Design review of the part built by this model. Coordinates are the model's own, in mm. A direction names the side the tool comes from. Give positions to 0.01 mm unless a question says otherwise; leave off trailing zeros. Order: outer loops, then holes, each group sorted by start corner. A loop starts at its lowest first (then second) coordinate and runs counter-clockwise, first axis right, second up. Notation, with made-up numbers: M 89.25,-26 L 99.25,-26 A14 ccw 99.25,0 Z; hole C 86.25,-30 d6. An arc over 180 degrees is marked long. Answer as a JSON object with one key per item and string values.
from build123d import *

# Parameters (mm, degrees)
SKETCH1_W            = 1094.236516538
SKETCH1_H            = 400
BOSS_EXTRUDE1_DEPTH  = 18
CAVITY1_START        = -15
CAVITY1_OUTLINE_W    = 18
CAVITY1_OUTLINE_H    = 18
CAVITY1_DEPTH        = 30
CAVITY1_START_2      = 813.236516538
CAVITY1_2_OUTLINE_W  = 18
CAVITY1_2_OUTLINE_H  = 18
CAVITY1_2_DEPTH      = 30
CAVITY1_START_3      = 389.118258269
CAVITY1_3_OUTLINE_W  = 18
CAVITY1_3_OUTLINE_H  = 18
CAVITY1_3_DEPTH      = 50
CAVITY1_START_4      = -35
CAVITY1_4_OUTLINE_W  = 18
CAVITY1_4_OUTLINE_H  = 18
CAVITY1_4_DEPTH      = 20
CAVITY1_START_5      = 15
CAVITY1_5_OUTLINE_W  = 18
CAVITY1_5_OUTLINE_H  = 18
CAVITY1_5_DEPTH      = 20
CAVITY1_START_6      = 793.236516538
CAVITY1_6_OUTLINE_W  = 18
CAVITY1_6_OUTLINE_H  = 18
CAVITY1_6_DEPTH      = 20
CAVITY1_START_7      = 843.236516538
CAVITY1_7_OUTLINE_W  = 18
CAVITY1_7_OUTLINE_H  = 18
CAVITY1_7_DEPTH      = 20
SKETCH2_W            = 18
SKETCH2_H            = 50
CUT_EXTRUDE1_DEPTH   = 987.255362837
SKETCH3_W            = 798.236516538
SKETCH3_H            = 209.4
CUT_EXTRUDE2_DEPTH   = 18
SKETCH4_W            = 734.236516538
SKETCH4_H            = 110.6
CUT_EXTRUDE3_DEPTH   = 20
M3_CLEARANCE_HOLE1_D = 3.4
SKETCH7_R            = 3
CUT_EXTRUDE4_DEPTH   = 30


# Read off the part's stored shape, not the designer's step: Cavity1
with BuildPart() as part:
    # Sketch1 → Boss-Extrude1 (new body)
    with BuildSketch(Plane.XY):
        with Locations((414.118258269, 20)):
            Rectangle(SKETCH1_W, SKETCH1_H)
    extrude(amount=BOSS_EXTRUDE1_DEPTH)

    # Cavity1 outline → Cavity1 (cut)
    with BuildSketch(Plane.YZ.offset(CAVITY1_START)):
        with Locations((-9, 9)):
            Rectangle(CAVITY1_OUTLINE_W, CAVITY1_OUTLINE_H)
        with Locations((-171, 9)):
            Rectangle(CAVITY1_OUTLINE_W, CAVITY1_OUTLINE_H)
    extrude(amount=CAVITY1_DEPTH, mode=Mode.SUBTRACT)

    # Cavity1 2 outline → Cavity1 2 (cut)
    with BuildSketch(Plane.YZ.offset(CAVITY1_START_2)):
        with Locations((-9, 9)):
            Rectangle(CAVITY1_2_OUTLINE_W, CAVITY1_2_OUTLINE_H)
        with Locations((-171, 9)):
            Rectangle(CAVITY1_2_OUTLINE_W, CAVITY1_2_OUTLINE_H)
    extrude(amount=CAVITY1_2_DEPTH, mode=Mode.SUBTRACT)

    # Cavity1 3 outline → Cavity1 3 (cut)
    with BuildSketch(Plane.YZ.offset(CAVITY1_START_3)):
        with Locations((-171, 9)):
            Rectangle(CAVITY1_3_OUTLINE_W, CAVITY1_3_OUTLINE_H)
    extrude(amount=CAVITY1_3_DEPTH, mode=Mode.SUBTRACT)

    # Cavity1 4 outline → Cavity1 4 (cut)
    with BuildSketch(Plane.YZ.offset(CAVITY1_START_4)):
        with Locations((-9, 9)):
            Rectangle(CAVITY1_4_OUTLINE_W, CAVITY1_4_OUTLINE_H)
    extrude(amount=CAVITY1_4_DEPTH, mode=Mode.SUBTRACT)

    # Cavity1 5 outline → Cavity1 5 (cut)
    with BuildSketch(Plane.YZ.offset(CAVITY1_START_5)):
        with Locations((-171, 9)):
            Rectangle(CAVITY1_5_OUTLINE_W, CAVITY1_5_OUTLINE_H)
    extrude(amount=CAVITY1_5_DEPTH, mode=Mode.SUBTRACT)

    # Cavity1 6 outline → Cavity1 6 (cut)
    with BuildSketch(Plane.YZ.offset(CAVITY1_START_6)):
        with Locations((-171, 9)):
            Rectangle(CAVITY1_6_OUTLINE_W, CAVITY1_6_OUTLINE_H)
    extrude(amount=CAVITY1_6_DEPTH, mode=Mode.SUBTRACT)

    # Cavity1 7 outline → Cavity1 7 (cut)
    with BuildSketch(Plane.YZ.offset(CAVITY1_START_7)):
        with Locations((-9, 9)):
            Rectangle(CAVITY1_7_OUTLINE_W, CAVITY1_7_OUTLINE_H)
    extrude(amount=CAVITY1_7_DEPTH, mode=Mode.SUBTRACT)

    # Sketch2 → Cut-Extrude1 (cut, through all)
    with BuildSketch(Plane.XY.offset(18)):
        with Locations((952.236516538, 145)):
            Rectangle(SKETCH2_W, SKETCH2_H)
        with Locations((952.236516538, -105)):
            Rectangle(SKETCH2_W, SKETCH2_H)
        with Locations((-124, -105)):
            Rectangle(SKETCH2_W, SKETCH2_H)
        with Locations((-124, 145)):
            Rectangle(SKETCH2_W, SKETCH2_H)
    extrude(amount=-CUT_EXTRUDE1_DEPTH, mode=Mode.SUBTRACT)

    # Sketch3 → Cut-Extrude2 (cut)
    with BuildSketch(Plane.XY.offset(18)):
        with Locations((414.118258269, 115.3)):
            Rectangle(SKETCH3_W, SKETCH3_H)
    extrude(amount=-CUT_EXTRUDE2_DEPTH, mode=Mode.SUBTRACT)

    # Sketch4 → Cut-Extrude3 (cut)
    with BuildSketch(Plane.XY.offset(18)):
        with Locations((414.118258269, -74.7)):
            Rectangle(SKETCH4_W, SKETCH4_H)
    extrude(amount=-CUT_EXTRUDE3_DEPTH, mode=Mode.SUBTRACT)

    # M3 Clearance Hole1 (through all)
    with Locations(Plane.XY.offset(18)):
        with Locations((-75, -9), (903.236516538, -9), (-75, -171), (212.059129134, -171), (616.177387403, -171), (893.236516538, -171), (952.236516538, -155), (952.236516538, 20), (952.236516538, 195), (-124, -155), (-124, 20), (-124, 195)):
            Hole(M3_CLEARANCE_HOLE1_D / 2)

    # Sketch7 → Cut-Extrude4 (cut)
    with BuildSketch(Plane.XY.offset(18)):
        with Locations((945.357836881, 122.121320344)):
            Circle(SKETCH7_R)
        with Locations((945.357836881, 167.878679656)):
            Circle(SKETCH7_R)
        with Locations((861.115196194, -15.878679656)):
            Circle(SKETCH7_R)
        with Locations((861.115196194, -2.121320344)):
            Circle(SKETCH7_R)
        with Locations((815.357836881, -2.121320344)):
            Circle(SKETCH7_R)
        with Locations((815.357836881, -15.878679656)):
            Circle(SKETCH7_R)
        with Locations((945.357836881, -127.878679656)):
            Circle(SKETCH7_R)
        with Locations((945.357836881, -82.121320344)):
            Circle(SKETCH7_R)
        with Locations((-117.121320344, 167.878679656)):
            Circle(SKETCH7_R)
        with Locations((-117.121320344, 122.121320344)):
            Circle(SKETCH7_R)
        with Locations((-117.121320344, -82.121320344)):
            Circle(SKETCH7_R)
        with Locations((-117.121320344, -127.878679656)):
            Circle(SKETCH7_R)
        with Locations((-32.878679656, -2.121320344)):
            Circle(SKETCH7_R)
        with Locations((-32.878679656, -15.878679656)):
            Circle(SKETCH7_R)
        with Locations((12.878679656, -15.878679656)):
            Circle(SKETCH7_R)
        with Locations((12.878679656, -2.121320344)):
            Circle(SKETCH7_R)
        with Locations((-15, -162)):
            Circle(SKETCH7_R)
        with Locations((35, -162)):
            Circle(SKETCH7_R)
        with Locations((793.236516538, -162)):
            Circle(SKETCH7_R)
        with Locations((843.236516538, -162)):
            Circle(SKETCH7_R)
        with Locations((389.116516538, -162)):
            Circle(SKETCH7_R)
        with Locations((439.116516538, -162)):
            Circle(SKETCH7_R)
    extrude(amount=-CUT_EXTRUDE4_DEPTH, mode=Mode.SUBTRACT)


solid = part.part
(1) We need section A-A (y = 69). Write out the cut boundary in (x, z).
Checked values:
{"outline": "M -133,0 L 15,0 L 15,18 L -133,18 Z; M 813.24,0 L 961.24,0 L 961.24,18 L 813.24,18 Z"}
(2) We need section C-C (z = 11.5). Count the separate pieces of the cut face and the enclosed holes in it, plus the area to 3 significant figures.
Checked values:
{"separate pieces": "1", "enclosed holes": "15", "area": "181,000 mm^2"}
(3) Draft analysis for pull direction X (two halves, no side actions). For faces 1 (the flat face through (961.237, 195, 9)), 2 (the flat face through (452, -9, 18)), 3 (the flat face through (838, -18, 9)), state which applies: +X half, -X half, draft (parallel to the pull), parting line (faces both ways), or undercut.
Checked values:
{"face 1": "+X half", "face 2": "draft", "face 3": "undercut"}
(4) We need section B-B (x = 101). Write out the cut boundary in (y, z).
Checked values:
{"outline": "M -180,0 L -130,0 L -130,18 L -180,18 Z; M -19.4,0 L 10.6,0 L 10.6,18 L -19.4,18 Z"}
(5) Tool access review of faces 4 (the flat face through (-115, 145, 9)), 5 (the flat face through (47, -75, 9)), 6 (the flat face through (-133, 19, 9)), 7 (the flat face through (414, -162, 9)): name each direction out of +Z, -Z, +X, -X, +Y, -Y from which nothing blocks a thin tool from reaching the whole face with its end or side.
Checked values:
{"face 4": "+Z, -Z, -X", "face 5": "+Z, -Z", "face 6": "+Z, -Z, -X, +Y, -Y", "face 7": "+Z, -Z, -Y"}
(6) To check wall thickness, follow L1, parallel to X at y = 195, z = 6; L2, parallel to X at y = -155, z = 13.25; L3, parallel to Y at x = 148, z = 2.25. State the ranges of each line that lie inside material, in increasing order. Write a range as from..to.
Checked values:
{"L1": "x = -133..-125.7, -122.3..15, 813.24..950.54, 953.94..961.24", "L2": "x = -133..-125.7, -122.3..950.54, 953.94..961.24", "L3": "y = -180..-130, -19.4..10.6"}
(7) Insertion check: pin 1 (4 mm diameter, centred on y = -121.5, z = 7.5, fed in from -X); pin 2 (8 mm diameter, centred on x = 832.5, z = 8.5, fed in from -Y); pin 3 (1 mm diameter, centred on x = 683.5, z = 4, fed in from +Y); pin 4 (5.5 mm diameter, centred on x = 843.24, y = -162, fed in from +Z). Each pin has a flat end and moves straight along its axis. Give the tip position at first contact, or say it passes through.
Checked values:
{"pin 1": "stops at x = -115", "pin 2": "stops at y = -162", "pin 3": "stops at y = 10.6", "pin 4": "passes through"}
